from build123d import *

# Parameters (mm, degrees)
CROQUIS1_W              = 76.2
CROQUIS1_H              = 101.6
SALIENTE_EXTRUIR1_DEPTH = 78.74
CROQUIS2_W              = 76.2
CROQUIS2_H              = 25.4
CORTAR_EXTRUIR1_DEPTH   = 96.52
CROQUIS3_W              = 76.2
CROQUIS3_H              = 38.1
CORTAR_EXTRUIR2_DEPTH   = 96.52
CROQUIS4_W              = 2
CROQUIS4_H              = 96.52
SALIENTE_EXTRUIR3_DEPTH = 73.66
CROQUIS6_W              = 96.52
CROQUIS6_H              = 17.379424015
CORTAR_EXTRUIR4_DEPTH   = 4
CORTAR_EXTRUIR5_DEPTH   = 4


with BuildPart() as part:
    # Croquis1 → Saliente-Extruir1 (new body)
    with BuildSketch(Plane(origin=(0, 0, 0), x_dir=(1, 0, 0), z_dir=(0, 1, 0))):
        Rectangle(CROQUIS1_W, CROQUIS1_H)
    extrude(amount=SALIENTE_EXTRUIR1_DEPTH)

    # Croquis2 → Cortar-Extruir1 (cut)
    with BuildSketch(Plane.XY.offset(50.8)):
        with Locations((0, 17.78)):
            Rectangle(CROQUIS2_W, CROQUIS2_H)
    extrude(amount=-CORTAR_EXTRUIR1_DEPTH, mode=Mode.SUBTRACT)

    # Croquis3 → Cortar-Extruir2 (cut)
    with BuildSketch(Plane.XY.offset(50.8)):
        with Locations((0, 54.61)):
            Rectangle(CROQUIS3_W, CROQUIS3_H)
    extrude(amount=-CORTAR_EXTRUIR2_DEPTH, mode=Mode.SUBTRACT)

    # Croquis4 → Saliente-Extruir3 (add, through all)
    with BuildSketch(Plane(origin=(0, 5.08, 0), x_dir=(1, 0, 0), z_dir=(0, 1, 0))):
        with Locations((-37.1, -2.54)):
            Rectangle(CROQUIS4_W, CROQUIS4_H)
    saliente_extruir3 = extrude(amount=SALIENTE_EXTRUIR3_DEPTH)

    # Croquis6 → Cortar-Extruir4 (cut)
    with BuildSketch(Plane.ZY.offset(38.1)):
        with Locations((2.54, 17.769712008)):
            Rectangle(CROQUIS6_W, CROQUIS6_H)
    cortar_extruir4 = extrude(amount=-CORTAR_EXTRUIR4_DEPTH, mode=Mode.SUBTRACT)

    # Croquis7 → Cortar-Extruir5 (cut)
    with BuildSketch(Plane.ZY.offset(38.1)):
        Polygon((50.8, 39.4956929), (-44.763376085, 39.4956929), (-45.72, 39.4956929), (-45.72, 69.66), (-44.763376085, 69.66), (50.8, 69.66), align=None)
    cortar_extruir5 = extrude(amount=-CORTAR_EXTRUIR5_DEPTH, mode=Mode.SUBTRACT)

    # Simetría1: Saliente-Extruir3, Cortar-Extruir4, Cortar-Extruir5 across plane
    add(saliente_extruir3.mirror(Plane(origin=(0, 0, 0), x_dir=(0, 0, 1), z_dir=(1, 0, 0))))
    add(cortar_extruir4.mirror(Plane(origin=(0, 0, 0), x_dir=(0, 0, 1), z_dir=(1, 0, 0))), mode=Mode.SUBTRACT)
    add(cortar_extruir5.mirror(Plane(origin=(0, 0, 0), x_dir=(0, 0, 1), z_dir=(1, 0, 0))), mode=Mode.SUBTRACT)


solid = part.part
Design review of the part built by this model. Coordinates are the model's own, in mm. A direction names the side the tool comes from. Round coordinates to 2 decimals unless told otherwise and drop trailing zeros. Order: outer loops, then holes, each group sorted by start corner. A loop starts at its lowest first (then second) coordinate and runs counter-clockwise, first axis right, second up. Notation, with made-up numbers: M -24.5,21 L -15.5,21 A11 ccw -15.5,29 Z; hole C 57,38.25 d6. An arc over 180 degrees is marked long. Answer as CSV lines item,"result". Start each with the question number.
1) For pin 1 Ø4 at (x, y) = (-13, 58) entering from +Z, flat-tipped, find the tip position at first contact; note if it passes through.
2) Wall thickness on line 1 along Y through (x, z) = (-14, 5); line 2 along X through (y, z) = (6.5, 22.5); line 3 along Z through (x, y) = (24.5, 26.5): over which ranges is each line inside the solid? List them lowest first. Write a range as [from, to].
3) Add section C-C (y = 52). Give the boundary of the cut face in (x, z), then the cut area to 3 significant figures.
4) The part is to be moulded in two halves that separate along Y. For faces 1 (the face through (36.1, 38, 3)), 2 (the face through (-1, 30.48, 3)), 3 (the face through (1, 2, 50.8)), 4 (the face through (-1, 78.74, -1)), say which applies: +Y half, -Y half, draft (parallel to the pull), parting line (faces both ways), or undercut.
5) Add section A-A (z = -19). Give the boundary of the cut face in (x, y).
6) Tool access review of faces 5 (the face through (-1, 5.08, 3)), 6 (the face through (-38.1, 39, 1)): name each direction out of +Z, -Z, +X, -X, +Y, -Y from which nothing blocks a thin tool from reaching the whole face with its end or side.
7) Add section B-B (x = 10). Give the boundary of the cut face in (y, z).
Resolved:
1,pin 1,"z = -45.72"
2,line 1,"[0, 5.08], [30.48, 35.56], [73.66, 78.74]"
2,line 2,"[-38.1, -36.1], [36.1, 38.1]"
2,line 3,"[-50.8, -45.72]"
3,outline,"M -38.1,-50.8 L 38.1,-50.8 L 38.1,-45.72 L -38.1,-45.72 Z"
3,area,"387 mm^2"
4,face 1,"undercut"
4,face 2,"undercut"
4,face 3,"draft"
4,face 4,"+Y half"
5,outline,"M -38.1,0 L 38.1,0 L 38.1,9.08 L 36.1,9.08 L 36.1,5.08 L -36.1,5.08 L -36.1,9.08 L -38.1,9.08 Z; M -38.1,26.46 L -36.1,26.46 L -36.1,30.48 L 36.1,30.48 L 36.1,26.46 L 38.1,26.46 L 38.1,39.5 L 36.1,39.5 L 36.1,35.56 L -36.1,35.56 L -36.1,39.5 L -38.1,39.5 Z; M -38.1,69.66 L -36.1,69.66 L -36.1,73.66 L 36.1,73.66 L 36.1,69.66 L 38.1,69.66 L 38.1,78.74 L -38.1,78.74 Z"
6,face 5,"+Z"
6,face 6,"+Z, -Z, -X, +Y, -Y"
7,outline,"M 0,-50.8 L 78.74,-50.8 L 78.74,50.8 L 73.66,50.8 L 73.66,-45.72 L 35.56,-45.72 L 35.56,50.8 L 30.48,50.8 L 30.48,-45.72 L 5.08,-45.72 L 5.08,50.8 L 0,50.8 Z"
